Could you check a few things on this model? Use its own coordinates, in mm. A direction names the side the tool comes from. Give positions to 0.01 mm unless a question says otherwise; leave off trailing zeros. Loops run counter-clockwise (first coordinate to the right, second up) from the corner with the lowest first, then second, coordinate; pieces in that order, holes last. Notation, with made-up numbers: (-9.75, -29.5) -> (11.25, -29.5) arc R9 ccw to (11.25, -21.5) -> close; hole circle Ø6 at (46.5, 58). An arc over 180 degrees is marked (long way). Put each result on its own line as item: value.
```python
from build123d import *

# Parameters (mm, degrees)
BOSS_EXTRUDE1_DEPTH = 50
CUT_EXTRUDE1_REACH  = 58.378
SKETCH2_R           = 2


with BuildPart() as part:
    # Sketch1 → Boss-Extrude1 (new body)
    with BuildSketch(Plane.XY):
        Polygon((0, 0), (-10, 0), (-35.357095704, -54.378467222), (-37.169711279, -53.533230699), (-11.274140522, 2), (0, 2), align=None)
    extrude(amount=BOSS_EXTRUDE1_DEPTH)

    # Sketch2 → Cut-Extrude1 (cut, up to next)
    with BuildSketch(Plane(origin=(0, 2, 0), x_dir=(1, 0, 0), z_dir=(0, 1, 0)), mode=Mode.PRIVATE) as cut_extrude1_sk1:
        with Locations((-5.637070261, -10)):
            Circle(SKETCH2_R)
    cut_extrude1_tool1 = extrude(cut_extrude1_sk1.sketch, amount=-CUT_EXTRUDE1_REACH, mode=Mode.PRIVATE) & part.part
    add(cut_extrude1_tool1.solids().sort_by_distance((-5.63707, 2, 10))[0], mode=Mode.SUBTRACT)
    # Sketch2 → Cut-Extrude1 (cut, up to next)
    with BuildSketch(Plane(origin=(0, 2, 0), x_dir=(1, 0, 0), z_dir=(0, 1, 0)), mode=Mode.PRIVATE) as cut_extrude1_sk2:
        with Locations((-5.637070261, -40)):
            Circle(SKETCH2_R)
    cut_extrude1_tool2 = extrude(cut_extrude1_sk2.sketch, amount=-CUT_EXTRUDE1_REACH, mode=Mode.PRIVATE) & part.part
    add(cut_extrude1_tool2.solids().sort_by_distance((-5.63707, 2, 40))[0], mode=Mode.SUBTRACT)


solid = part.part
```
1. Thinking about a two-plate mould opening in Z: for faces 1 (the face through (-6.071, 1.014, 41.952)), 2 (the face through (0, 1, 25)), 3 (the face through (-21, -22, 50)), 4 (the face through (-7.11, 1.01, 8.65)), which applies, pulls with the +Z half, pulls with the -Z half, needs draft (parallel to the pull), parting line crosses it, or undercut?
Recorded:
face 1: undercut
face 2: needs draft
face 3: pulls with the +Z half
face 4: undercut
2. If we section it at A-A (z = 10): List the corners of the cut face in (x, y) for me.
Recorded:
outline: (-37.17, -53.53) -> (-35.36, -54.38) -> (-10, 0) -> (-7.64, 0) -> (-7.64, 2) -> (-11.27, 2) -> close; (-3.64, 0) -> (0, 0) -> (0, 2) -> (-3.64, 2) -> close
3. For faces 5 (the face through (-5, 0, 25)), 6 (the face through (-6, 2, 25)), which set-ups out of +Z, -Z, +X, -X, +Y, -Y let a thin tool reach every point of the face, with its end or its side?
Recorded:
face 5: +Z, -Z, +X, -Y
face 6: +Z, -Z, +X, -X, +Y
4. If we section it at D-D (y = -48.5): List the corners of the cut face in (x, z) for me.
Recorded:
outline: (-34.82, 0) -> (-32.62, 0) -> (-32.62, 50) -> (-34.82, 50) -> close
5. If we section it at C-C (x = -2.5): List the corners of the cut face in (y, z) for me.
Recorded:
outline: (0, 0) -> (2, 0) -> (2, 50) -> (0, 50) -> close
6. I need wall thicknesses on line 1 (Y direction, x = -4.5, z = 46.5); line 2 (X direction, y = 0.9, z = 40); line 3 (X direction, y = -5.5, z = 20). Which ranges of each line are inside material? Lowest first, please.
Recorded:
line 1: y = 0 to 2
line 2: x = -11.79 to -7.64, -3.64 to 0
line 3: x = -14.77 to -12.56
7. If we section it at B-B (z = 19): List the corners of the cut face in (x, y) for me, then the cut area to 3 significant figures.
Recorded:
outline: (-37.17, -53.53) -> (-35.36, -54.38) -> (-10, 0) -> (0, 0) -> (0, 2) -> (-11.27, 2) -> close
area: 143 mm^2
8. I'm going to push flat-ended pins straight in: pin 1 (5 mm diameter, centred on x = -5.64, z = 10, fed in from -Y); pin 2 (12 mm diameter, centred on x = -23.5, y = -38, fed in from +Z); pin 3 (1.5 mm diameter, centred on y = -36, z = 37.5, fed in from -X); pin 4 (11 mm diameter, centred on x = -5.5, z = 30, fed in from -Y). Where does each tip first touch, or does it pass through?
Recorded:
pin 1: stops at y = 0
pin 2: stops at z = 50
pin 3: stops at x = -29.34
pin 4: stops at y = -2.14
